Design review of the part built by this model. Coordinates are the model's own, in mm. Face numbers are marked on the shaded views. A direction names the side the tool comes from. Coordinates: 2 decimals unless noted, no trailing zeros. Loops run counter-clockwise (first coordinate to the right, second up) from the corner with the lowest first, then second, coordinate; pieces in that order, holes last. Notation, with made-up numbers: (63, 71.5) - (85, 71.5) arc R36 cw to (85, 106.5) - close; hole circle Ø9 at (23.5, -9). An arc over 180 degrees is marked (long way). Answer in a Markdown table with one row per item. Add a question column.
(1) We need section A-A, the plane z = -12.5. Write out the cut boundary in (x, y).
(2) We need section C-C, the plane y = 0.5. Write out the cut boundary in (x, z).
(3) We need section B-B, the plane x = -5.5. Write out the cut boundary in (y, z).
(4) We need section D-D, the plane y = 6.25. Write out the cut boundary in (x, z).
(5) For the marked faces 4 and 5, list the 3-axis set-ups (+Z, -Z, +X, -X, +Y, -Y) from which the entire face can be reached by the end or side of a thin tool; tool diameter is ignored.
(6) To check wall thickness, follow L1, parallel to Z at x = -4.75, y = 1.75; L2, parallel to Z at x = -9.75, y = 3; L3, parallel to Y at x = -21.75, z = 16. State the ranges of each line that lie inside material, in increasing order. Write a range as [from, to].
(7) Clearance check with flat-ended pins moving along their axes: pin 1 (1.1 mm diameter, centred on x = -20.5, z = -11, fed in from +Y); pin 2 (1.5 mm diameter, centred on x = -15, z = -7.5, fed in from -Y); pin 3 (1.7 mm diameter, centred on y = 3.5, z = -11, fed in from -X); pin 4 (1.5 mm diameter, centred on x = -10.5, y = 6, fed in from -Z). State where each tip first meets the part, or that it passes through.
(8) The part is to be moulded in two halves that separate along X. For the marked faces 1, 2 and 3, say which applies: released by +X, released by -X, zero draft, split by the parting line, or undercut.
from build123d import *

# Parameters (mm, degrees)
SKETCH1_W           = 24
SKETCH1_H           = 40
BOSS_EXTRUDE1_DEPTH = 5
SKETCH2_W           = 1
SKETCH2_H           = 1.5
BOSS_EXTRUDE2_DEPTH = 4
SKETCH4_R           = 3.5
BOSS_EXTRUDE4_DEPTH = 9


with BuildPart() as part:
    # Sketch1 → Boss-Extrude1 (new body)
    with BuildSketch(Plane(origin=(0, 0, 0), x_dir=(1, 0, 0), z_dir=(0, 1, 0))):
        with Locations((-12, -10.571428571)):
            Rectangle(SKETCH1_W, SKETCH1_H)
    extrude(amount=BOSS_EXTRUDE1_DEPTH)

    # Sketch2 → Boss-Extrude2 (add)
    with BuildSketch(Plane(origin=(0, 0, -9.428571429), x_dir=(-1, 0, 0), z_dir=(0, 0, -1))):
        with Locations((3.5, 3.479518838)):
            Rectangle(SKETCH2_W, SKETCH2_H)
        with Locations((7.5, 3.479518838)):
            Rectangle(SKETCH2_W, SKETCH2_H)
        with Locations((16.5, 3.479518838)):
            Rectangle(SKETCH2_W, SKETCH2_H)
        with Locations((20.5, 3.479518838)):
            Rectangle(SKETCH2_W, SKETCH2_H)
    extrude(amount=BOSS_EXTRUDE2_DEPTH)

    # Sketch4 → Boss-Extrude4 (add)
    with BuildSketch(Plane(origin=(0, 0, -13.428571429), x_dir=(-1, 0, 0), z_dir=(0, 0, -1))):
        with Locations((5.5, 3.40608753)):
            Circle(SKETCH4_R)
        with Locations((18.5, 3.40608753)):
            Circle(SKETCH4_R)
    extrude(amount=BOSS_EXTRUDE4_DEPTH)


solid = part.part
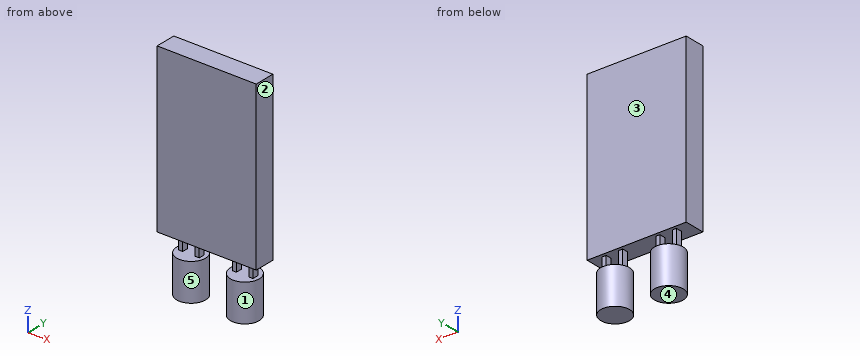
Responses:
| question | item | result |
|---|---|---|
| 1 | outline | (-21, 2.73) - (-20, 2.73) - (-20, 4.23) - (-21, 4.23) - close; (-17, 2.73) - (-16, 2.73) - (-16, 4.23) - (-17, 4.23) - close; (-8, 2.73) - (-7, 2.73) - (-7, 4.23) - (-8, 4.23) - close; (-4, 2.73) - (-3, 2.73) - (-3, 4.23) - (-4, 4.23) - close |
| 2 | outline | (-24, -9.43) - (0, -9.43) - (0, 30.57) - (-24, 30.57) - close; (-20.45, -22.43) - (-16.55, -22.43) - (-16.55, -13.43) - (-20.45, -13.43) - close; (-7.45, -22.43) - (-3.55, -22.43) - (-3.55, -13.43) - (-7.45, -13.43) - close |
| 3 | outline | (-0.09, -22.43) - (6.91, -22.43) - (6.91, -13.43) - (-0.09, -13.43) - close; (0, -9.43) - (5, -9.43) - (5, 30.57) - (0, 30.57) - close |
| 4 | outline | (-20.54, -22.43) - (-16.46, -22.43) - (-16.46, -13.43) - (-20.54, -13.43) - close; (-7.54, -22.43) - (-3.46, -22.43) - (-3.46, -13.43) - (-7.54, -13.43) - close |
| 5 | face 4 | -Z, +X, -X, +Y, -Y |
| 5 | face 5 | -Z |
| 6 | L1 | z = [-22.43, -13.43], [-9.43, 30.57] |
| 6 | L2 | z = [-9.43, 30.57] |
| 6 | L3 | y = [0, 5] |
| 7 | pin 1 | stops at y = 4.23 |
| 7 | pin 2 | stops at y = 0 |
| 7 | pin 3 | stops at x = -21 |
| 7 | pin 4 | passes through |
| 8 | face 1 | undercut |
| 8 | face 2 | released by +X |
| 8 | face 3 | zero draft |
